from build123d import *

# Parameters (mm, degrees)
BOSS_EXTRUDE1_DEPTH = 150
SKETCH2_R           = 26.75
SKETCH2_R_2         = 2.2
CUT_EXTRUDE1_DEPTH  = 3.175
CUT_EXTRUDE2_REACH  = 184.942
SKETCH3_R           = 2


with BuildPart() as part:
    # Sketch1 → Boss-Extrude1 (new body)
    with BuildSketch(Plane.XY):
        Polygon((0, 78.463366337), (25.4, 78.463366337), (25.4, -23.136633663), (0, -23.136633663), (0, -19.961633663), (22.225, -19.961633663), (22.225, 75.288366337), (0, 75.288366337), align=None)
    extrude(amount=BOSS_EXTRUDE1_DEPTH)

    # Sketch2 → Cut-Extrude1 (cut)
    with BuildSketch(Plane(origin=(25.4, 0, 0), x_dir=(0, 0, -1), z_dir=(1, 0, 0))):
        with Locations(Location((-75, 16.863366337, 0), (0, 0, 90))):
            Circle(SKETCH2_R)
        with Locations(Location((-75, 47.863366337, 0), (0, 0, 90))):
            Circle(SKETCH2_R_2)
        with Locations(Location((-53.079689783, 38.783676553, 0), (0, 0, 90))):
            Circle(SKETCH2_R_2)
        with Locations(Location((-44, 16.863366337, 0), (0, 0, 90))):
            Circle(SKETCH2_R_2)
        with Locations(Location((-53.079689783, -5.05694388, 0), (0, 0, 90))):
            Circle(SKETCH2_R_2)
        with Locations(Location((-75, -14.136633663, 0), (0, 0, 90))):
            Circle(SKETCH2_R_2)
        with Locations(Location((-96.920310217, -5.05694388, 0), (0, 0, 90))):
            Circle(SKETCH2_R_2)
        with Locations(Location((-106, 16.863366337, 0), (0, 0, 90))):
            Circle(SKETCH2_R_2)
        with Locations(Location((-96.920310217, 38.783676553, 0), (0, 0, 90))):
            Circle(SKETCH2_R_2)
    extrude(amount=-CUT_EXTRUDE1_DEPTH, mode=Mode.SUBTRACT)

    # Cut-Extrude2: up to this face of the body (flat: up to its plane)
    cut_extrude2_end = Plane(part.part.faces().sort_by_distance((12.7, -23.136633663, 75))[0])
    # Sketch3 → Cut-Extrude2 (cut, up to the picked face)
    with BuildSketch(Plane(origin=(0, 78.463366337, 0), x_dir=(1, 0, 0), z_dir=(0, 1, 0)), mode=Mode.PRIVATE) as cut_extrude2_sk1:
        with Locations(Location((12.7, -75, 0), (0, 0, 270))):
            Circle(SKETCH3_R)
    cut_extrude2_tool1 = split(extrude(cut_extrude2_sk1.sketch, amount=-CUT_EXTRUDE2_REACH, mode=Mode.PRIVATE), bisect_by=cut_extrude2_end, keep=Keep.BOTH, mode=Mode.PRIVATE)
    # Sketch3 → Cut-Extrude2 (cut, up to the picked face)
    with BuildSketch(Plane(origin=(0, 78.463366337, 0), x_dir=(1, 0, 0), z_dir=(0, 1, 0)), mode=Mode.PRIVATE) as cut_extrude2_sk2:
        with Locations(Location((12.7, -105, 0), (0, 0, 270))):
            Circle(SKETCH3_R)
    cut_extrude2_tool2 = split(extrude(cut_extrude2_sk2.sketch, amount=-CUT_EXTRUDE2_REACH, mode=Mode.PRIVATE), bisect_by=cut_extrude2_end, keep=Keep.BOTH, mode=Mode.PRIVATE)
    # Sketch3 → Cut-Extrude2 (cut, up to the picked face)
    with BuildSketch(Plane(origin=(0, 78.463366337, 0), x_dir=(1, 0, 0), z_dir=(0, 1, 0)), mode=Mode.PRIVATE) as cut_extrude2_sk3:
        with Locations(Location((12.7, -135, 0), (0, 0, 270))):
            Circle(SKETCH3_R)
    cut_extrude2_tool3 = split(extrude(cut_extrude2_sk3.sketch, amount=-CUT_EXTRUDE2_REACH, mode=Mode.PRIVATE), bisect_by=cut_extrude2_end, keep=Keep.BOTH, mode=Mode.PRIVATE)
    # Sketch3 → Cut-Extrude2 (cut, up to the picked face)
    with BuildSketch(Plane(origin=(0, 78.463366337, 0), x_dir=(1, 0, 0), z_dir=(0, 1, 0)), mode=Mode.PRIVATE) as cut_extrude2_sk4:
        with Locations(Location((12.7, -45, 0), (0, 0, 270))):
            Circle(SKETCH3_R)
    cut_extrude2_tool4 = split(extrude(cut_extrude2_sk4.sketch, amount=-CUT_EXTRUDE2_REACH, mode=Mode.PRIVATE), bisect_by=cut_extrude2_end, keep=Keep.BOTH, mode=Mode.PRIVATE)
    # Sketch3 → Cut-Extrude2 (cut, up to the picked face)
    with BuildSketch(Plane(origin=(0, 78.463366337, 0), x_dir=(1, 0, 0), z_dir=(0, 1, 0)), mode=Mode.PRIVATE) as cut_extrude2_sk5:
        with Locations(Location((12.7, -15, 0), (0, 0, 270))):
            Circle(SKETCH3_R)
    cut_extrude2_tool5 = split(extrude(cut_extrude2_sk5.sketch, amount=-CUT_EXTRUDE2_REACH, mode=Mode.PRIVATE), bisect_by=cut_extrude2_end, keep=Keep.BOTH, mode=Mode.PRIVATE)
    add(cut_extrude2_tool1.solids().sort_by(Axis((12.7, 78.463366, 75), (0, -1, 0)))[0], mode=Mode.SUBTRACT)
    add(cut_extrude2_tool2.solids().sort_by(Axis((12.7, 78.463366, 105), (0, -1, 0)))[0], mode=Mode.SUBTRACT)
    add(cut_extrude2_tool3.solids().sort_by(Axis((12.7, 78.463366, 135), (0, -1, 0)))[0], mode=Mode.SUBTRACT)
    add(cut_extrude2_tool4.solids().sort_by(Axis((12.7, 78.463366, 45), (0, -1, 0)))[0], mode=Mode.SUBTRACT)
    add(cut_extrude2_tool5.solids().sort_by(Axis((12.7, 78.463366, 15), (0, -1, 0)))[0], mode=Mode.SUBTRACT)


solid = part.part
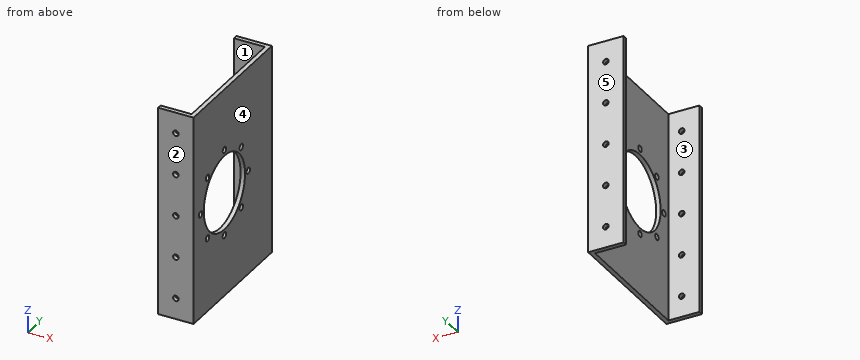
Could you check a few things on this model? Use its own coordinates, in mm. Face numbers are marked on the shaded views. A direction names the side the tool comes from. Coordinates: 2 decimals unless noted, no trailing zeros. Loops run counter-clockwise (first coordinate to the right, second up) from the corner with the lowest first, then second, coordinate; pieces in that order, holes last.
1. We'd pull the mould along Y, two halves only. Please class the marked faces 3, 4 and 5: released by +Y, released by -Y, zero draft, split by the parting line, or undercut.
2. For P1, Ø2.5, axis at y = -5.06, z = 53.08, coming from the +X side; P2, Ø2, axis at y = 45, z = 78.5, coming from the -X side (3 decimals), each with a flat end and sliding along its axis, tell me the tip position at first contact or that it passes through.
3. Imagine slicing it at D-D (x = 12.7). Give the number of separate pieces and of enclosed holes in the cut face, and give its area (4 significant figures).
4. Imagine slicing it at B-B (z = 75). Please give me the cut outline in (x, y) (3 decimals).
5. For the marked faces 1 and 2, which set-ups out of +Z, -Z, +X, -X, +Y, -Y let a thin tool reach every point of the face, with its end or its side?
6. I need wall thicknesses on L1, parallel to Y at x = 19.5, z = 140; L2, parallel to X at y = 76.2, z = 135; L3, parallel to X at y = -2, z = 56 (3 decimals). Which ranges of each line are inside material? Lowest first, please.
7. Imagine slicing it at A-A (x = 20.5). Please give me the cut outline in (y, z), and give its area (4 significant figures).
8. Imagine slicing it at C-C (y = 0.5). Please give me the cut outline in (x, z) (3 decimals), and give its area (3 significant figures).
Computed values:
1. face 3: undercut
1. face 4: zero draft
1. face 5: released by +Y
2. P1: passes through
2. P2: stops at x = 22.225
3. separate pieces: 12
3. enclosed holes: 0
3. area: 825.5 mm2
4. outline: (0, -23.137) - (10.7, -23.137) - (10.7, -19.962) - (0, -19.962) - close; (0, 75.288) - (10.7, 75.288) - (10.7, 78.463) - (0, 78.463) - close; (14.7, -23.137) - (25.4, -23.137) - (25.4, -16.337) - (22.225, -16.337) - (22.225, -19.962) - (14.7, -19.962) - close; (14.7, 75.288) - (22.225, 75.288) - (22.225, 50.063) - (25.4, 50.063) - (25.4, 78.463) - (14.7, 78.463) - close; (22.225, -11.937) - (25.4, -11.937) - (25.4, -9.887) - (22.225, -9.887) - close; (22.225, 43.613) - (25.4, 43.613) - (25.4, 45.663) - (22.225, 45.663) - close
5. face 1: +Z, -Z, -X
5. face 2: +Z, -Z, +X, -X, -Y
6. L1: y = -23.14 to -19.96, 75.29 to 78.46
6. L2: x = 0 to 10.7, 14.7 to 25.4
6. L3: x = 22.225 to 25.4
7. outline: (-23.14, 0) - (-19.96, 0) - (-19.96, 150) - (-23.14, 150) - close; (75.29, 0) - (78.46, 0) - (78.46, 150) - (75.29, 150) - close
7. area: 952.5 mm2
8. outline: (22.225, 0) - (25.4, 0) - (25.4, 53.839) - (22.225, 53.839) - close; (22.225, 96.161) - (25.4, 96.161) - (25.4, 150) - (22.225, 150) - close
8. area: 342 mm2
